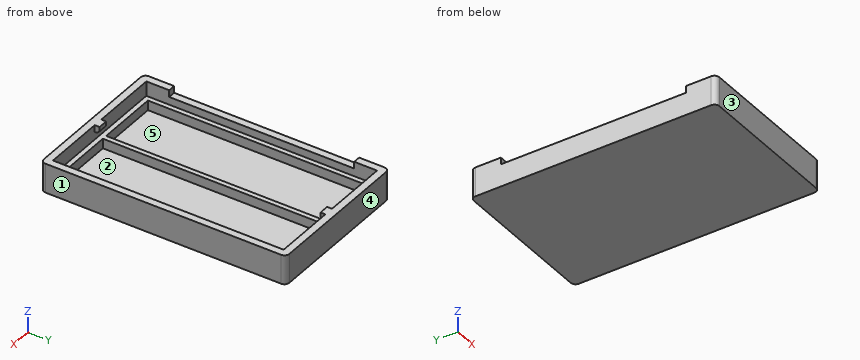
```python
from build123d import *

# Parameters (mm, degrees)
SKETCH1_W           = 47.4
SKETCH1_H           = 28.4
BOSS_EXTRUDE1_DEPTH = 1
SKETCH2_W           = 31.4
SKETCH2_H           = 50.4
SKETCH2_W_2         = 28.4
SKETCH2_H_2         = 47.4
BOSS_EXTRUDE2_DEPTH = 6
SKETCH3_W           = 28.4
SKETCH3_H           = 47.4
SKETCH3_W_2         = 12.7
SKETCH3_H_2         = 45.4
BOSS_EXTRUDE3_DEPTH = 2
SKETCH4_W           = 2
SKETCH4_H           = 1
BOSS_EXTRUDE4_DEPTH = 1.4
CHAMFER1_SIZE       = 0.5
CUT_EXTRUDE1_START  = -1.4
SKETCH5_W           = 9.609138978
SKETCH5_H           = 38
CUT_EXTRUDE1_DEPTH  = 1.4
FILLET1_R           = 1


with BuildPart() as part:
    # Sketch1 → Boss-Extrude1 (new body)
    with BuildSketch(Plane(origin=(0, 0, 0), x_dir=(0, 1, 0), z_dir=(0, 0, 1))):
        Rectangle(SKETCH1_W, SKETCH1_H)
    extrude(amount=BOSS_EXTRUDE1_DEPTH)



with BuildPart() as body_2:
    # Sketch2 → Boss-Extrude2 (new body)
    with BuildSketch(Plane(origin=(0, 0, 0), x_dir=(1, 0, 0), z_dir=(0, 0, -1))):
        Rectangle(SKETCH2_W, SKETCH2_H)
        Rectangle(SKETCH2_W_2, SKETCH2_H_2, mode=Mode.SUBTRACT)
    extrude(amount=-BOSS_EXTRUDE2_DEPTH)


with BuildPart() as part_1:
    add(part.part)

    add(body_2.part)  # Boss-Extrude3 merges body 2
    # Sketch3 → Boss-Extrude3 (add)
    with BuildSketch(Plane.XY.offset(1)):
        Rectangle(SKETCH3_W, SKETCH3_H)
        with Locations((-6.85, 0)):
            Rectangle(SKETCH3_W_2, SKETCH3_H_2, mode=Mode.SUBTRACT)
        with Locations((6.85, 0)):
            Rectangle(SKETCH3_W_2, SKETCH3_H_2, mode=Mode.SUBTRACT)
    extrude(amount=BOSS_EXTRUDE3_DEPTH)

    # Sketch4 → Boss-Extrude4 (add)
    with BuildSketch(Plane.XY.offset(4.6)):
        with Locations((0.5, 23.2)):
            Rectangle(SKETCH4_W, SKETCH4_H)
        with Locations((0.5, -23.2)):
            Rectangle(SKETCH4_W, SKETCH4_H)
    extrude(amount=BOSS_EXTRUDE4_DEPTH)

    # Chamfer1
    chamfer1_edges = [part_1.edges().sort_by_distance(p)[0] for p in [
        (0.5, 22.7, 4.6),
        (0.5, -22.7, 4.6),
    ]]
    chamfer(chamfer1_edges, length=CHAMFER1_SIZE)

    # Sketch5 → Cut-Extrude1 (cut)
    with BuildSketch(Plane.XY.offset(6).offset(CUT_EXTRUDE1_START)):
        with Locations((-14.2, 0)):
            Rectangle(SKETCH5_W, SKETCH5_H)
    extrude(amount=CUT_EXTRUDE1_DEPTH, mode=Mode.SUBTRACT)

    # Fillet1
    fillet1_edges = [part_1.edges().sort_by_distance(p)[0] for p in [
        (-15.7, -25.2, 3),
        (15.7, -25.2, 3),
        (15.7, 25.2, 3),
        (-15.7, 25.2, 3),
    ]]
    fillet(fillet1_edges, radius=FILLET1_R)


solid = part_1.part
```
Check sheet for the modelled part. Datum: model origin and axes. Units: mm. Face numbers are marked on the shaded views. A direction names the side the tool comes from. Round coordinates to 2 decimals unless told otherwise and drop trailing zeros. Loops run counter-clockwise (first coordinate to the right, second up) from the corner with the lowest first, then second, coordinate; pieces in that order, holes last. Notation, with made-up numbers: (36.25, 77) -> (48.25, 77) arc R31 cw to (48.25, 104) -> close; hole circle Ø9 at (30.25, -39.75). An arc over 180 degrees is marked (long way). Write item = value, one per line. Start each with the question number.
1) Gauge pin test, flat ends, axial feed: pin 1 Ø1.5 at (x, z) = (-15, 5.5) entering from +Y; pin 2 Ø2 at (x, y) = (10, 0.5) entering from +Z; pin 3 Ø10 at (x, y) = (2.5, -6) entering from +Z. Record the tip position at first contact, or that the pin passes through.
2) Set-up check for the marked faces 4 and 5: record each of +Z, -Z, +X, -X, +Y, -Y from which the full face is reachable in a straight line by a thin tool's end or side.
3) Sectioned sample at C-C, the plane x = 4. Record the cut outline in (y, z), plus the area to 3 significant figures.
4) Thickness scan on probe 1 along X at (y, z) = (16, 2.45); probe 2 along Y at (x, z) = (4, 1.15); probe 3 along X at (y, z) = (-17.5, 4.2). Record the ranges inside material, lowest first.
5) Sectioned sample at A-A, the plane z = 1.9. Record the cut outline in (x, y).
6) Sectioned sample at D-D, the plane y = -21. Record the cut outline in (x, z).
7) Release check for a two-part mould opening along Y. For the marked faces 1, 2 and 3 record: released by +Y, released by -Y, zero draft, split by the parting line, or undercut.
8) Sectioned sample at B-B, the plane y = 10.5. Record the cut outline in (x, z).
Results are:
q1.pin_1 = 25.2
q1.pin_2 = 1
q1.pin_3 = 3
q2.face_4 = +Z, -Z, +X, -X, +Y
q2.face_5 = +Z
q3.outline = (-25.2, 0) -> (25.2, 0) -> (25.2, 6) -> (23.7, 6) -> (23.7, 3) -> (22.7, 3) -> (22.7, 1) -> (-22.7, 1) -> (-22.7, 3) -> (-23.7, 3) -> (-23.7, 6) -> (-25.2, 6) -> close
q3.area = 69.4 mm^2
q4.probe_1 = -15.7 to -13.2, -0.5 to 0.5, 13.2 to 15.7
q4.probe_2 = -25.2 to -22.7, 22.7 to 25.2
q4.probe_3 = -15.7 to -14.2, 14.2 to 15.7
q5.outline = (-15.7, -24.2) arc R1 ccw to (-14.7, -25.2) -> (14.7, -25.2) arc R1 ccw to (15.7, -24.2) -> (15.7, 24.2) arc R1 ccw to (14.7, 25.2) -> (-14.7, 25.2) arc R1 ccw to (-15.7, 24.2) -> close; hole (-13.2, -22.7) -> (-0.5, -22.7) -> (-0.5, 22.7) -> (-13.2, 22.7) -> close; hole (0.5, -22.7) -> (13.2, -22.7) -> (13.2, 22.7) -> (0.5, 22.7) -> close
q6.outline = (-15.7, 0) -> (15.7, 0) -> (15.7, 6) -> (14.2, 6) -> (14.2, 3) -> (13.2, 3) -> (13.2, 1) -> (0.5, 1) -> (0.5, 3) -> (-0.5, 3) -> (-0.5, 1) -> (-13.2, 1) -> (-13.2, 3) -> (-14.2, 3) -> (-14.2, 6) -> (-15.7, 6) -> close
q7.face_1 = zero draft
q7.face_2 = undercut
q7.face_3 = released by -Y
q8.outline = (-15.7, 0) -> (15.7, 0) -> (15.7, 6) -> (14.2, 6) -> (14.2, 3) -> (13.2, 3) -> (13.2, 1) -> (0.5, 1) -> (0.5, 3) -> (-0.5, 3) -> (-0.5, 1) -> (-13.2, 1) -> (-13.2, 3) -> (-14.2, 3) -> (-14.2, 4.6) -> (-15.7, 4.6) -> close
